from build123d import *

# Parameters (mm, degrees)
SKETCH1_R           = 17
BOSS_EXTRUDE2_DEPTH = 18
SKETCH3_R           = 2.75
CUT_EXTRUDE2_DEPTH  = 64
SKETCH4_R           = 4
CUT_EXTRUDE3_DEPTH  = 5
SKETCH5_RX          = 17
SKETCH5_RY          = 17
BOSS_EXTRUDE3_DEPTH = 0.5
SKETCH6_R           = 4
CUT_EXTRUDE4_DEPTH  = 0.5


with BuildPart() as part:
    # Sketch1 → Boss-Extrude2 (new body)
    with BuildSketch(Plane(origin=(0, 0, 0), x_dir=(1, 0, 0), z_dir=(0, 1, 0))):
        with Locations(Location((0, 0, 0), (0, 0, 270))):
            Circle(SKETCH1_R)
    extrude(amount=BOSS_EXTRUDE2_DEPTH)

    # Sketch3 → Cut-Extrude2 (cut)
    with BuildSketch(Plane(origin=(0, 18, 0), x_dir=(1, 0, 0), z_dir=(0, 1, 0))):
        with Locations(Location((0, 0, 0), (0, 0, 270))):
            Circle(SKETCH3_R)
    extrude(amount=-CUT_EXTRUDE2_DEPTH, mode=Mode.SUBTRACT)

    # Sketch4 → Cut-Extrude3 (cut)
    with BuildSketch(Plane(origin=(0, 18, 0), x_dir=(1, 0, 0), z_dir=(0, 1, 0))):
        with Locations(Location((0, 0, 0), (0, 0, 270))):
            Circle(SKETCH4_R)
    extrude(amount=-CUT_EXTRUDE3_DEPTH, mode=Mode.SUBTRACT)

    # Sketch5 → Boss-Extrude3 (add)
    with BuildSketch(Plane(origin=(0, 18, 0), x_dir=(1, 0, 0), z_dir=(0, 1, 0))):
        with Locations(Location((0, 0), (0, 0, -2.815048359))):
            Ellipse(SKETCH5_RX, SKETCH5_RY)
    extrude(amount=BOSS_EXTRUDE3_DEPTH)

    # Sketch6 → Cut-Extrude4 (cut)
    with BuildSketch(Plane(origin=(0, 18.5, 0), x_dir=(1, 0, 0), z_dir=(0, 1, 0))):
        with Locations(Location((0, 0, 0), (0, 0, 270))):
            Circle(SKETCH6_R)
    extrude(amount=-CUT_EXTRUDE4_DEPTH, mode=Mode.SUBTRACT)


solid = part.part
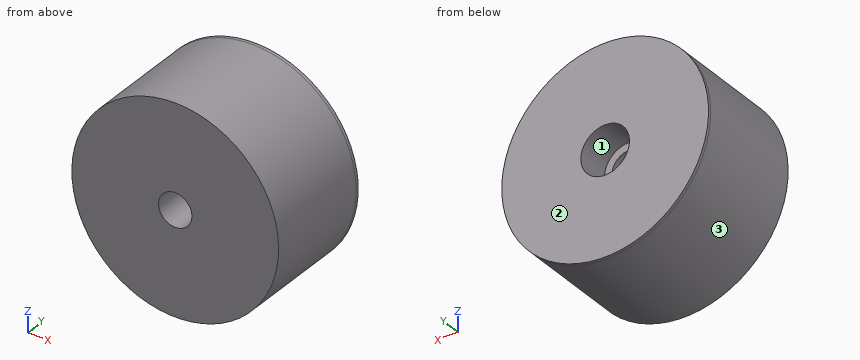
Read the model definition and answer for the solid it produces. Units are mm, in the model's axes. Face numbers are marked on the shaded views. Coordinates: 2 decimals unless noted, no trailing zeros. Order: outer loops, then holes, each group sorted by start corner. A loop starts at its lowest first (then second) coordinate and runs counter-clockwise, first axis right, second up. Notation, with made-up numbers: (37, -39.75) -> (61, -39.75) arc R24 cw to (61, -20.75) -> close; hole circle Ø2 at (-10.5, 88.25). An arc over 180 degrees is marked (long way). Answer as a JSON object with one key per item and string values.
1) The mould has two halves that part along X. Classify the marked faces 1, 2 and 3: released by +X, released by -X, zero draft, split by the parting line, or undercut.
Model answer:
{"face 1": "undercut", "face 2": "zero draft", "face 3": "split by the parting line"}
2) A cutting plane is placed at B-B, the plane y = 16.25. Determine the outline of the cut face in (x, z).
Model answer:
{"outline": "circle Ø34 at (0, 0); hole circle Ø8 at (0, 0)"}
3) A cutting plane is placed at A-A, the plane y = 9.5. Determine the outline of the cut face in (x, z), plus the area to 3 significant figures.
Model answer:
{"outline": "circle Ø34 at (0, 0); hole circle Ø5.5 at (0, 0)", "area": "884 mm²"}
4) Consider line 1 along X through (y, z) = (5, 0); line 2 along X through (y, z) = (14.9, 0); line 3 along Z through (x, y) = (3, 14). Determine where each line is inside the solid, lowest interval first. Write a range as from..to.
Model answer:
{"line 1": "x = -17..-2.75, 2.75..17", "line 2": "x = -17..-4, 4..17", "line 3": "z = -16.73..-2.65, 2.65..16.73"}
5) Each of these flat-tipped pins is pushed along its axis until it touches: pin 1 (3.5 mm diameter, centred on x = 0, z = 0, fed in from -Y); pin 2 (6.5 mm diameter, centred on x = 0.5, z = 0.5, fed in from +Y); pin 3 (2 mm diameter, centred on y = 6, z = 12, fed in from +X); pin 4 (4 mm diameter, centred on x = -6.5, y = 5.5, fed in from -Z). Where does it stop, or does it pass through?
Model answer:
{"pin 1": "passes through", "pin 2": "stops at y = 13", "pin 3": "stops at x = 12.96", "pin 4": "stops at z = -16.39"}
